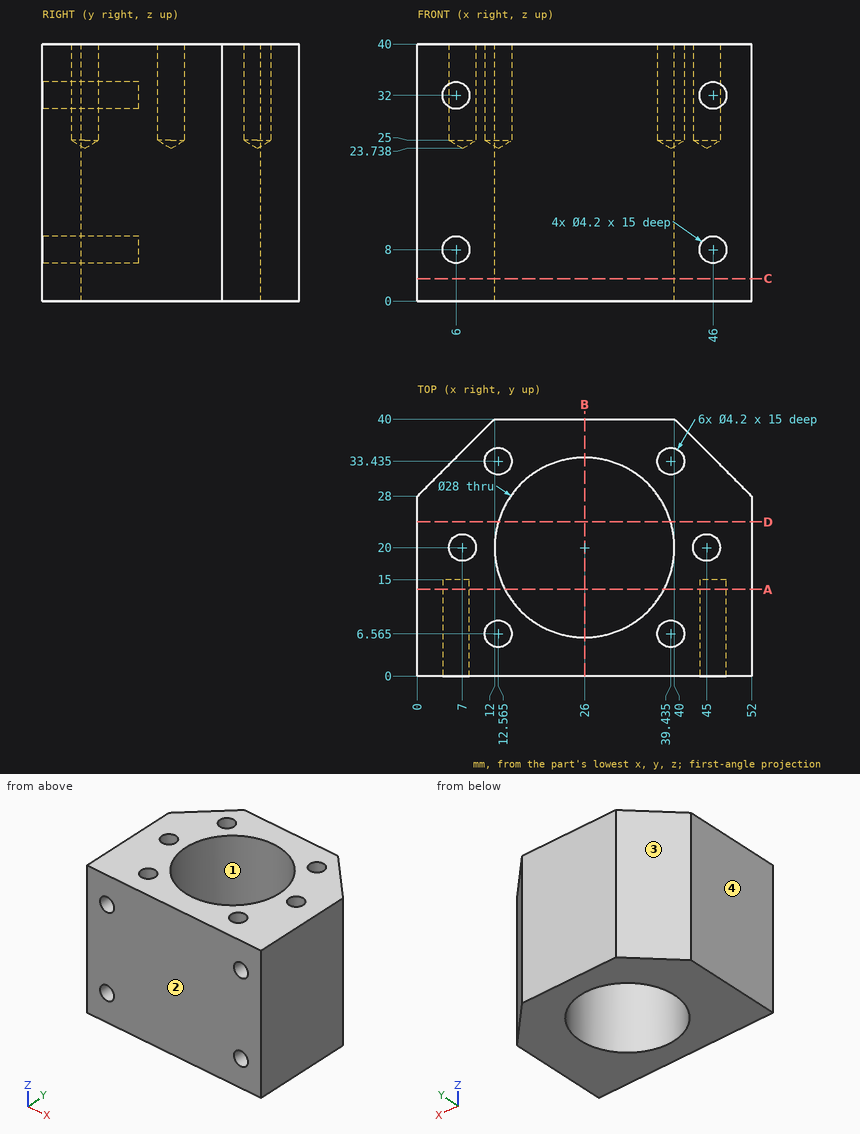
Geometry check sheet. Reference: drawing and pictorial views, mm from the part's lowest x, y, z. Round coordinates to 2 decimals unless told otherwise and drop trailing zeros. Loops run counter-clockwise (first coordinate to the right, second up) from the corner with the lowest first, then second, coordinate; pieces in that order, holes last. Notation, with made-up numbers: (27, -40) - (60, -40) arc R22 ccw to (60, -26) - close; hole circle Ø5 at (73.25, 45.25). An arc over 180 degrees is marked (long way). Answer in a Markdown table with one row per item. Add a question column.
Q1. Material ranges on line 1 (X direction, y = 4, z = 32); line 2 (X direction, y = 32, z = 30); line 3 (X direction, y = 7.5, z = 32) (1 decimal), recorded low to high.
Q2. Release check for a two-part mould opening along Y. For the marked faces 1, 2, 3 and 4 record: pulls with the +Y half, pulls with the -Y half, needs draft (parallel to the pull), parting line crosses it, or undercut.
Q3. Section check C-C on z = 3.5. Enter the section's corners in (x, y), plus the area to 3 significant figures.
Q4. Section check A-A on y = 13.5. Enter the section's corners in (x, z), plus the area to 3 significant figures.
Q5. Section check D-D on y = 24. Enter the section's corners in (x, z).
Q6. Gauge pin test, flat ends, axial feed: pin 1 (1 mm diameter, centred on y = 31.5, z = 28, fed in from -X); pin 2 (1 mm diameter, centred on y = 30, z = 34, fed in from -X); pin 3 (1.3 mm diameter, centred on x = 6, z = 32.5, fed in from -Y). Record the tip position at first contact, or that the pin passes through.
Q7. Section check B-B on x = 26. Enter the section's corners in (y, z), plus the area to 3 significant figures.
Found:
| question | item | result |
|---|---|---|
| 1 | line 1 | x = 0 to 3.9, 8.1 to 43.9, 48.1 to 52 |
| 1 | line 2 | x = 4 to 11.03, 14.1 to 18.79, 33.21 to 37.9, 40.97 to 48 |
| 1 | line 3 | x = 0 to 3.9, 8.1 to 10.7, 14.4 to 19.7, 32.3 to 37.6, 41.3 to 43.9, 48.1 to 52 |
| 2 | face 1 | undercut |
| 2 | face 2 | pulls with the -Y half |
| 2 | face 3 | pulls with the +Y half |
| 2 | face 4 | needs draft |
| 3 | outline | (0, 0) - (52, 0) - (52, 28) - (40, 40) - (12, 40) - (0, 28) - close; hole circle Ø28 at (26, 20) |
| 3 | area | 1,320 mm² |
| 4 | outline | (0, 0) - (13.6, 0) - (13.6, 40) - (0, 40) - close; (38.4, 0) - (52, 0) - (52, 40) - (38.4, 40) - close; hole circle Ø4.2 at (6, 8); hole circle Ø4.2 at (6, 32); hole circle Ø4.2 at (46, 8); hole circle Ø4.2 at (46, 32) |
| 4 | area | 1,030 mm² |
| 5 | outline | (0, 0) - (12.58, 0) - (12.58, 40) - (0, 40) - close; (39.42, 0) - (52, 0) - (52, 40) - (39.42, 40) - close |
| 6 | pin 1 | stops at x = 3 |
| 6 | pin 2 | stops at x = 1.5 |
| 6 | pin 3 | stops at y = 15 |
| 7 | outline | (0, 0) - (6, 0) - (6, 40) - (0, 40) - close; (34, 0) - (40, 0) - (40, 40) - (34, 40) - close |
| 7 | area | 480 mm² |
